The listing builds one solid part. Answer for the finished solid, in the listing's coordinates (mm). A direction names the side the tool comes from. Coordinates: 2 decimals unless noted, no trailing zeros. Order: outer loops, then holes, each group sorted by start corner. A loop starts at its lowest first (then second) coordinate and runs counter-clockwise, first axis right, second up. Notation, with made-up numbers: (22.5, 23.25) -> (27.5, 23.25) arc R25 ccw to (27.5, 42.25) -> close; hole circle Ø10 at (-26.5, 36.5). An arc over 180 degrees is marked (long way). Return JSON: item names as keys, results as strings.
```python
from build123d import *

# Parameters (mm, degrees)
F1_DEPTH = 88.9
F3_DEPTH = 5
F4_W     = 81.28
F4_H     = 7.62
F5_DEPTH = 7.62
F6_R     = 3.81
F7_R     = 2.54
F8_SIZE  = 7.61999


# Not quite as in the source:
# - a fillet or chamfer is up to 0.001 mm smaller than in the source, because OpenCascade refuses the exact size


with BuildPart() as f1:
    # F0 (on Right) → F1 (new body)
    with BuildSketch(Plane.YZ):
        Polygon((17.24, 2), (17.24, 0), (59.88, 0), (59.88, 21.8881247946), (25.3046089437, 30.7845262293), (24.6716719012, 28.3246500739), (57.88, 19.78), (57.88, 2), align=None)
        Polygon((-25.4, 21.8881247946), (-25.4, 0), (17.24, 0), (17.24, 2), (-23.4, 2), (-23.4, 19.78), (9.8083280988, 28.3246500739), (9.1753910563, 30.7845262293), align=None)
    extrude(amount=F1_DEPTH)

    # F2 (on Right) → F3 (join)
    with BuildSketch(Plane.YZ):
        Polygon((33.83, 2), (38.83, 2), (38.83, 17.7), (38.83, 24.6816494725), (33.83, 25.9681716437), (33.83, 17.7), align=None)
        Polygon((-4.35, 17.7), (-4.35, 2), (0.65, 2), (0.65, 17.7), (0.65, 25.9681716437), (-4.35, 24.6816494725), align=None)
    extrude(amount=F3_DEPTH)

    # F4 (on face) → F5 (join)
    with BuildSketch(Plane.YZ.offset(88.9)):
        with Locations((17.24, 5.81)):
            Rectangle(F4_W, F4_H)
    extrude(amount=-F5_DEPTH)

    # F6
    f6_edges = [f1.edges().sort_by_distance(p)[0] for p in [
        (44.45, -25.4, 0),
        (44.45, 59.88, 0),
        (44.45, -25.4, 21.888125),
        (44.45, 59.88, 21.888125),
    ]]
    fillet(f6_edges, radius=F6_R)

    # F7
    f7_edges = [f1.edges().sort_by_distance(p)[0] for p in [
        (40.64, 57.88, 2),
        (40.64, -23.4, 2),
        (44.45, -23.4, 19.78),
        (44.45, 57.88, 19.78),
    ]]
    fillet(f7_edges, radius=F7_R)

    # F8 (size 7.62 in the source; OpenCascade refuses exactly that, so slightly less here)
    f8_edges = [f1.edges().sort_by_distance(p)[0] for p in [
        (81.28, 17.24, 9.62),
    ]]
    chamfer(f8_edges, length=F8_SIZE)


solid = f1.part
```
Item 1: Flat-ended cylindrical pins translate along their axes: pin 1 (2 mm diameter, centred on x = 17, z = 22, fed in from +Y); pin 2 (1 mm diameter, centred on x = 41.5, y = 23, fed in from +Z). Find the tip coordinate at first contact, or state that the pin passes through.
Answer list:
{"pin 1": "y = 59.27", "pin 2": "z = 2"}
Item 2: Determine the mould class of faces 1 (the flat face through (5, 36, 14)), 2 (the flat face through (88.9, 17, 9)), 3 (the flat face through (43.828, 40.103, 24.354)) for opening direction X: pulls with the +X half, pulls with the -X half, needs draft (parallel to the pull), parting line crosses it, or undercut.
Answer list:
{"face 1": "undercut", "face 2": "pulls with the +X half", "face 3": "needs draft"}
Item 3: The part is cut by section A-A on z = 14.5. Determine the outline of the cut face in (x, y), plus the area to 3 significant figures.
Answer list:
{"outline": "(0, -25.4) -> (88.9, -25.4) -> (88.9, -23.4) -> (0, -23.4) -> close; (0, -4.35) -> (5, -4.35) -> (5, 0.65) -> (0, 0.65) -> close; (0, 33.83) -> (5, 33.83) -> (5, 38.83) -> (0, 38.83) -> close; (0, 57.88) -> (88.9, 57.88) -> (88.9, 59.88) -> (0, 59.88) -> close", "area": "406 mm2"}
Item 4: The part is cut by section C-C on z = 27. Determine the outline of the cut face in (x, y), plus the area to 3 significant figures.
Answer list:
{"outline": "(0, -5.53) -> (88.9, -5.53) -> (88.9, 4.66) -> (0, 4.66) -> close; (0, 29.82) -> (88.9, 29.82) -> (88.9, 40.01) -> (0, 40.01) -> close", "area": "1,810 mm2"}
Item 5: Which of the six approach directions +Z, -Z, +X, -X, +Y, -Y give full straight-line access (tool end or side, diameter ignored) to faces 4 (the flat face through (43.828, 9.496, 29.537)), 5 (the flat face through (5, -2, 14)), 6 (the flat face through (44, -23.4, 11))?
Answer list:
{"face 4": "+Z, +X, -X", "face 5": "none", "face 6": "-X"}
Item 6: The part is cut by section B-B on x = 76. Determine the outline of the cut face in (y, z).
Answer list:
{"outline": "(-25.4, 3.81) arc R3.81 ccw to (-21.59, 0) -> (56.07, 0) arc R3.81 ccw to (59.88, 3.81) -> (59.88, 18.93) arc R3.81 ccw to (57.02, 22.62) -> (25.3, 30.78) -> (24.67, 28.32) -> (55.97, 20.27) arc R2.54 cw to (57.88, 17.81) -> (57.88, 4.54) arc R2.54 cw to (55.34, 2) -> (-20.86, 2) arc R2.54 cw to (-23.4, 4.54) -> (-23.4, 17.81) arc R2.54 cw to (-21.49, 20.27) -> (9.81, 28.32) -> (9.18, 30.78) -> (-22.54, 22.62) arc R3.81 ccw to (-25.4, 18.93) -> close"}
Item 7: Find the intervals of material crossed by probe 1 along Y at (x, z) = (19.5, 16); probe 2 along Y at (x, z) = (84, 3.5); probe 3 along Z at (x, y) = (76.5, 17), in increasing order.
Answer list:
{"probe 1": "-25.4 to -23.4, 57.88 to 59.88", "probe 2": "-25.39 to 59.87", "probe 3": "0 to 2"}
